The model under review builds one solid part; all positions refer to its coordinate system, in mm. Give positions to 0.01 mm unless a question says otherwise; leave off trailing zeros. Order: outer loops, then holes, each group sorted by start corner. A loop starts at its lowest first (then second) coordinate and runs counter-clockwise, first axis right, second up. Notation, with made-up numbers: (-38, -26.5) - (15, -26.5) arc R9 cw to (15, -22.5) - close; hole circle Ø2 at (53.25, 42). An arc over 180 degrees is marked (long way). Use a Markdown table: item, result. Add a question column.
Autodesk Inventor part; units mm, degrees
ref_plane "YZ Plane" through (0, 0, 0) normal (1, 0, 0) x (0, 1, 0)
ref_plane "XZ Plane" through (0, 0, 0) normal (0, 1, 0) x (-1, 0, 0)
ref_plane "XY Plane" through (0, 0, 0) normal (0, 0, 1) x (1, 0, 0)
sketch "Sketch1" plane through (0, 0, 0) normal (0, 1, 0) x (-1, 0, 0)
  circle A0 centre (0, 0) radius 2.6
  line L0 (0, 0) -> (0, -2.6) construction
  line L1 (0, 0) -> (-2.6, 0) construction
  circle A1 centre (0, -20) radius 2.6
  circle A2 centre (-20, 0) radius 2.6
  circle A3 centre (-20, -20) radius 2.6
  circle A4 centre (0, 108) radius 2.6
  circle A5 centre (-20, 108) radius 2.6
  circle A6 centre (0, 128) radius 2.6
  circle A7 centre (-20, 128) radius 2.6
  circle A8 centre (20, 54) radius 19.15
  circle A9 centre (43.57, 30.43) radius 2.6
  circle A10 centre (-3.57, 30.43) radius 2.6
  circle A11 centre (-3.57, 77.57) radius 2.6
  circle A12 centre (43.57, 77.57) radius 2.6
  circle A13 centre (43.57, 77.57) radius 5.775 construction
  circle A14 centre (43.57, 30.43) radius 5.775 construction
  circle A15 centre (0, 128) radius 8.95 construction
  circle A16 centre (-20, 128) radius 8.95 construction
  circle A17 centre (0, -20) radius 8.95 construction
  circle A18 centre (-20, -20) radius 8.95 construction
  line L2 (7.0435, 133.5219) -> (48.1148, 81.133)
  line L3 (48.1148, 26.867) -> (7.0435, -25.5219)
  line L4 (0, 136.95) -> (-20, 136.95)
  line L5 (-28.95, 128) -> (-28.95, -20)
  line L6 (-20, -28.95) -> (0, -28.95)
  line L7 (49.345, 77.57) -> (49.345, 30.43)
  arc A19 (49.345, 77.57) -> (48.1148, 81.133) centre (43.57, 77.57) ccw
  arc A20 (48.1148, 26.867) -> (49.345, 30.43) centre (43.57, 30.43) ccw
  arc A21 (0, -28.95) -> (7.0435, -25.5219) centre (0, -20) ccw
  arc A22 (-28.95, -20) -> (-20, -28.95) centre (-20, -20) ccw
  arc A23 (-20, 136.95) -> (-28.95, 128) centre (-20, 128) ccw
  arc A24 (7.0435, 133.5219) -> (0, 136.95) centre (0, 128) ccw
  point P0 (0, -22.6)
  point P1 (-2.6, -20)
  point P2 (-20, -2.6)
  point P3 (-22.6, 0)
  point P4 (-20, -22.6)
  point P5 (-22.6, -20)
  dimension "d0" = 5.2
  dimension "d3" = 20
  dimension "d6" = 20
  dimension "d9" = 108
  dimension "d10" = 20
  dimension "d11" = 20
  dimension "d13" = 54
  dimension "d14" = 38.3
  dimension "d15" = 23.57
  dimension "d16" = 23.57
  dimension "d17" = 47.14
  dimension "d18" = 47.14
  dimension "d19" = 3.175
  dimension "d20" = 6.35
extrude "Extrusion1" add sketch "Sketch1" along normal blind 4.7625
equation "\"d18\" = d17"
properties part number "CNC-000-StructureGusset1" material "Steel AISI 1008 91 HR"
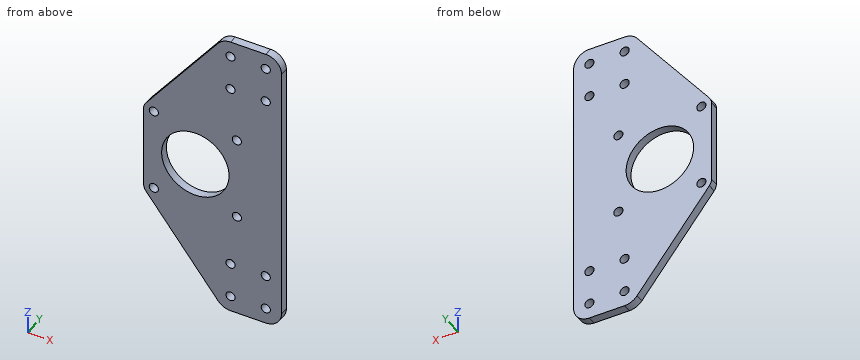
Q1. Wall thickness on probe 1 along Z at (x, y) = (0, 2.4); probe 2 along Z at (x, y) = (3.57, 3.6): over which ranges is each line inside the solid? List them lowest first.
Q2. We need section D-D (x = -12). Write out the cut boundary in (y, z), plus the area to 4 significant figures.
Q3. We need section B-B (x = -43.57). Write out the cut boundary in (y, z).
Q4. We need section C-C (y = 2.8). Count the separate pieces of the cut face and the enclosed holes in it, plus the area to 3 significant figures.
Q5. Clearance check with a flat-ended pin moving along its axis: P1, Ø3, axis at x = 20, z = 108, coming from the -Y side. State where the tip first meets the part, or that it passes through.
Here are the results:
| question | item | result |
|---|---|---|
| 1 | probe 1 | -28.95 to -22.6, -17.4 to -2.6, 2.6 to 105.4, 110.6 to 125.4, 130.6 to 136.95 |
| 1 | probe 2 | -28.95 to 27.83, 33.03 to 74.97, 80.17 to 136.95 |
| 2 | outline | (0, -19.2) - (4.76, -19.2) - (4.76, 36.6) - (0, 36.6) - close; (0, 71.4) - (4.76, 71.4) - (4.76, 127.2) - (0, 127.2) - close |
| 2 | area | 531.5 mm2 |
| 3 | outline | (0, 21.07) - (4.76, 21.07) - (4.76, 27.83) - (0, 27.83) - close; (0, 33.03) - (4.76, 33.03) - (4.76, 74.97) - (0, 74.97) - close; (0, 80.17) - (4.76, 80.17) - (4.76, 86.93) - (0, 86.93) - close |
| 4 | separate pieces | 1 |
| 4 | enclosed holes | 13 |
| 4 | area | 8,960 mm2 |
| 5 | P1 | through |
